from build123d import *

# Parameters (mm, degrees)
PAD_DEPTH       = 12
POCKET_DEPTH    = 1
SKETCH003_R     = 8
POCKET001_DEPTH = 12.001
SKETCH004_W     = 180
SKETCH004_H     = 18
PAD001_DEPTH    = 18


with BuildPart() as part:
    # Sketch → Pad (new body)
    with BuildSketch(Plane.XY):
        Polygon((0, 0), (0, 140), (160, 140), (160, -140), (0, -140), align=None)
    extrude(amount=PAD_DEPTH)

    # Sketch002 (on Face7 of Pad) → Pocket (cut)
    with BuildSketch(Plane.XY.offset(12)):
        Polygon((0, -140), (0, -71.973152), (160, -140), align=None)
    extrude(amount=-POCKET_DEPTH, mode=Mode.SUBTRACT)

    # Sketch003 (on Face5 of Pocket) → Pocket001 (cut, through all)
    with BuildSketch(Plane.XY.offset(12)):
        with Locations((60, 37.5)):
            Circle(SKETCH003_R)
        with Locations((135, 37.5)):
            Circle(SKETCH003_R)
        with Locations((135, -37.5)):
            Circle(SKETCH003_R)
        with Locations((60, -37.5)):
            Circle(SKETCH003_R)
    extrude(amount=-POCKET001_DEPTH, mode=Mode.SUBTRACT)

    # Sketch004 (on Face4 of Pocket001) → Pad001 (join)
    with BuildSketch(Plane(origin=(0, 0, 0), x_dir=(1, 0, 0), z_dir=(0, 0, -1))):
        with Locations((90, 109)):
            Rectangle(SKETCH004_W, SKETCH004_H)
        with Locations((90, -109)):
            Rectangle(SKETCH004_W, SKETCH004_H)
    extrude(amount=PAD001_DEPTH)


solid = part.part
The listing builds one solid part. Answer for the finished solid, in the listing's coordinates (mm). A direction names the side the tool comes from. Coordinates: 2 decimals unless noted, no trailing zeros. Write each loop counter-clockwise with the first axis right and the second up, starting at its lowest first coordinate (ties: lowest second). Pieces come first, ordered by that corner, then holes. Notation, with made-up numbers: (-4, 81.25) - (19, 81.25) arc R16 cw to (19, 97.25) - close; hole circle Ø5 at (60.5, 21.5). An arc over 180 degrees is marked (long way). Put each result on its own line as item: value.
1. The part is cut by section D-D on x = 13.5. Give the vertices of the cut face in (y, z), plus the area to 3 significant figures.
Answer sheet:
outline: (-140, 0) - (-118, 0) - (-118, -18) - (-100, -18) - (-100, 0) - (100, 0) - (100, -18) - (118, -18) - (118, 0) - (140, 0) - (140, 12) - (-77.71, 12) - (-77.71, 11) - (-140, 11) - close
area: 3,950 mm^2
2. Find the intervals of material crossed by line 1 along Y through (x, z) = (135, 5.25); line 2 along Y through (x, z) = (79.5, -13.25); line 3 along Z through (x, y) = (77, 71), in increasing order. Write a range as from..to.
Answer sheet:
line 1: y = -140..-45.5, -29.5..29.5, 45.5..140
line 2: y = -118..-100, 100..118
line 3: z = 0..12
3. The part is cut by section B-B on z = -7.75. Give the vertices of the cut face in (x, y), plus the area to 3 significant figures.
Answer sheet:
outline: (0, -118) - (180, -118) - (180, -100) - (0, -100) - close; (0, 100) - (180, 100) - (180, 118) - (0, 118) - close
area: 6,480 mm^2
4. Flat-ended cylindrical pins translate along their axes: pin 1 Ø10 at (y, z) = (88, 3) entering from +X; pin 2 Ø14.5 at (x, y) = (172, -111.5) entering from +Z; pin 3 Ø14.5 at (x, z) = (79, -11) entering from +Y; pin 4 Ø14.5 at (x, y) = (60, 37.5) entering from -Z. Find the tip coordinate at first contact, or state that the pin passes through.
Answer sheet:
pin 1: stops at x = 160
pin 2: stops at z = 0
pin 3: stops at y = 118
pin 4: passes through
5. The part is cut by section A-A on y = 37.5. Give the vertices of the cut face in (x, z), plus the area to 3 significant figures.
Answer sheet:
outline: (0, 0) - (52, 0) - (52, 12) - (0, 12) - close; (68, 0) - (127, 0) - (127, 12) - (68, 12) - close; (143, 0) - (160, 0) - (160, 12) - (143, 12) - close
area: 1,540 mm^2
6. The part is cut by section C-C on x = 60. Give the vertices of the cut face in (y, z).
Answer sheet:
outline: (-140, 0) - (-118, 0) - (-118, -18) - (-100, -18) - (-100, 0) - (-45.5, 0) - (-45.5, 12) - (-97.48, 12) - (-97.48, 11) - (-140, 11) - close; (-29.5, 0) - (29.5, 0) - (29.5, 12) - (-29.5, 12) - close; (45.5, 0) - (100, 0) - (100, -18) - (118, -18) - (118, 0) - (140, 0) - (140, 12) - (45.5, 12) - close
7. A tool of negligible diameter and unlimited length cuts with its end or side. For faces 1 (the face through (89, 118, -9)), 2 (the face through (46, -121, 11)), 3 (the face through (81, 1, 0)), 4 (the face through (89, -118, -9)), from which of +Z, -Z, +X, -X, +Y, -Y can it reach the whole face along a straight path? Write none if from no direction.
Answer sheet:
face 1: -Z, +X, -X, +Y
face 2: +Z, -X, -Y
face 3: -Z, +X, -X
face 4: -Z, +X, -X, -Y
8. Determine the mould class of faces 5 (the face through (170, -109, 0)), 6 (the face through (0, 2, 7)), 7 (the face through (142.63, 39.9, 6.08)) for opening direction X: pulls with the +X half, pulls with the -X half, needs draft (parallel to the pull), parting line crosses it, or undercut.
Answer sheet:
face 5: needs draft
face 6: pulls with the -X half
face 7: undercut
